Autodesk Fusion 360 part; units mm, degrees
sketch "Schizzo8" plane through (0, 0, 0) normal (0, 1, 0) x (1, 0, 0)
  line L0 (45.3365, 90.3085) -> (91.8565, 90.3085)
  line L1 (91.8565, 90.3085) -> (91.8565, 66.9085)
  line L2 (91.8565, 66.9085) -> (45.3365, 66.9085)
  line L3 (45.3365, 66.9085) -> (45.3365, 90.3085)
  circle A0 centre (45.3365, 90.3085) radius 2.75
  circle A1 centre (91.8565, 90.3085) radius 2.75
  circle A2 centre (91.8565, 66.9085) radius 2.75
  circle A3 centre (45.3365, 66.9085) radius 2.75
  line L4 (45.3365, 90.3085) -> (47.3365, 90.3085)
  line L5 (45.3365, 90.3085) -> (43.3365, 90.3085)
  line L6 (43.3365, 90.3085) -> (43.3365, 66.9085)
  line L7 (47.3365, 90.3085) -> (47.3365, 66.9085)
  line L8 (91.8565, 90.3085) -> (93.8565, 90.3085)
  line L9 (91.8565, 90.3085) -> (89.8565, 90.3085)
  line L10 (89.8565, 90.3085) -> (89.8565, 66.9085)
  line L11 (93.8565, 90.3085) -> (93.8565, 66.9085)
  line L12 (93.8565, 78.6085) -> (93.8565, 80.6085)
  line L13 (93.8565, 78.6085) -> (93.8565, 76.6085)
  line L14 (93.8565, 80.6085) -> (43.3365, 80.6085)
  line L15 (93.8565, 76.6085) -> (43.3365, 76.6085)
  dimension "d71" = 46.52
  dimension "d72" = 23.4
  dimension "d73" = 5.5
  dimension "d74" = 5.5
  dimension "d75" = 5.5
  dimension "d76" = 5.5
  dimension "d77" = 2
  dimension "d78" = 2
  dimension "d79" = 2
  dimension "d80" = 2
  dimension "d81" = 2
  dimension "d82" = 2
extrude "Estrusione14" add sketch "Schizzo8" along normal blind 4 contours L3 A0 L7 L14 | L3 A0 L6 L14 | L3 L7 L14 L15 | L3 L6 L14 L15 | L7 L10 L14 L15 | L3 A3 L7 L15 | L3 A3 L6 L15 | L1 A1 L10 L14 | L1 L10 L14 L15 | L1 A1 L11 L14 | L1 A2 L10 L15 | L1 L11 L12 L13 L14 L15 | L1 A2 L11 L15
extrude "Estrusione15" add sketch "Schizzo8" along normal blind 30 contours L0 A0 L4 L5 L6 | L0 L3 A0 L4 L7 | L3 A0 L5 L6 | L0 A0 L7 | L0 A1 L8 L9 L11 | L0 A1 L10 | L0 L1 A1 L9 L10 | L2 L3 A3 L7 | L2 L3 A3 | L1 A1 L8 L11 | L2 A3 L7 | L2 A2 L10 | L1 L2 A2 L10 | L1 L2 A2
hole "Foratura5" at (45.3365, 30, -90.3085) direction (0, -1, 0) diameter 2.5 depth 7 tip angle 118
hole "Foratura6" at (45.3365, 30, -66.9085) direction (0, -1, 0) diameter 2.5 depth 7 tip angle 118
hole "Foratura7" at (91.8565, 30, -66.9085) direction (0, -1, 0) diameter 2.5 depth 7 tip angle 118
hole "Foratura8" at (91.8565, 30, -90.3085) direction (0, -1, 0) diameter 2.5 depth 7 tip angle 118
Part model, mm, in its own coordinate system. A direction names the side the tool comes from. Coordinates: 2 decimals unless noted, no trailing zeros. Order: outer loops, then holes, each group sorted by start corner. A loop starts at its lowest first (then second) coordinate and runs counter-clockwise, first axis right, second up. Notation, with made-up numbers: M 22.25,6 L 29.25,6 A23 cw 29.25,16 Z; hole C 18.5,-10 d4. An arc over 180 degrees is marked long. One line per question, with ' | ' between items.
Q1. Two-plate mould, pull along X, no slides. Class faces 4 (the face through (67, 0, -80)), 5 (the face through (43.336, 2, -79)), 6 (the face through (89.856, 2, -85)): +X half, -X half, draft (parallel to the pull), parting line (faces both ways), or undercut.
A:
face 4: draft | face 5: -X half | face 6: undercut
Q2. 3-axis set-ups, long thin cutter, end or side, ignore diameter. For faces 1 (the face through (92, 30, -92)), 2 (the face through (44.1, 26.5, -90.5)), 3 (the face through (47.336, 2, -73)): which of +Z, -Z, +X, -X, +Y, -Y reach the whole face in a straight line?
A:
face 1: +Z, -Z, +X, -X, +Y | face 2: +Y | face 3: +Y, -Y
Q3. Slice it at B-B (y = 27.75). Give the cut face in (x, z).
A:
outline: C 45.34,-90.31 d5.5; C 45.34,-66.91 d5.5; C 91.86,-90.31 d5.5; C 91.86,-66.91 d5.5; hole C 45.34,-90.31 d2.5; hole C 45.34,-66.91 d2.5; hole C 91.86,-90.31 d2.5; hole C 91.86,-66.91 d2.5
Q4. Slice it at A-A (z = -72.5). Give the cut face in (x, y), and give its area (3 significant figures).
A:
outline: M 43.34,0 L 47.34,0 L 47.34,4 L 43.34,4 Z; M 89.86,0 L 93.86,0 L 93.86,4 L 89.86,4 Z | area: 32.0 mm^2
Q5. Pin check, flat tips, straight feed: P1, Ø1.2, axis at y = 2, z = -73.5, coming from the -X side; P2, Ø6, axis at x = 71.5, z = -71, coming from the +Y side; P3, Ø4.5, axis at y = 2.5, z = -83, coming from the +X side; P4, Ø3, axis at x = 45.34, z = -66.91, coming from the +Y side. Stop position of each tip, or through.
A:
P1: stops at x = 43.34 | P2: passes through | P3: stops at x = 93.86 | P4: stops at y = 30
Q6. Slice it at D-D (x = 75.5). Give the cut face in (y, z).
A:
outline: M 0,-80.61 L 4,-80.61 L 4,-76.61 L 0,-76.61 Z
Q7. Slice it at C-C (y = 20.75). Give the cut face in (x, z), and give its area (3 significant figures).
A:
outline: C 45.34,-90.31 d5.5; C 45.34,-66.91 d5.5; C 91.86,-90.31 d5.5; C 91.86,-66.91 d5.5 | area: 95.0 mm^2
Q8. Drill centre lines: line 1 (Z direction, x = 45.5, y = 25); line 2 (Y direction, x = 71.5, z = -77.5); line 3 (X direction, y = 18, z = -66.5). Where is each one in solid material? Low to high.
A:
line 1: z = -93.05 to -91.55, -89.07 to -87.56, -69.65 to -68.15, -65.67 to -64.16 | line 2: y = 0 to 4 | line 3: x = 42.62 to 48.06, 89.14 to 94.58
